```python
from build123d import *

# Parameters (mm, degrees)
F0_W     = 40
F0_H     = 61
F1_DEPTH = 2
F0_H_2   = 19
F2_DEPTH = 25
F3_R     = 8.5
F4_DEPTH = 17
F5_R     = 19.99999


# Not quite as in the source:
# - a fillet or chamfer is up to 0.001 mm smaller than in the source, because OpenCascade refuses the exact size


with BuildPart() as f1:
    # F0 (on Top) → F1 (new body)
    with BuildSketch(Plane.XY):
        with Locations((-2.8480109572, 28.6193176061)):
            Rectangle(F0_W, F0_H)
    extrude(amount=F1_DEPTH)

    # F0 (on Top) → F2 (join)
    with BuildSketch(Plane.XY):
        with Locations((-2.8480109572, -11.3806823939)):
            Rectangle(F0_W, F0_H_2)
    extrude(amount=F2_DEPTH)

    # F3 (on face) → F4 (cut)
    with BuildSketch(Plane(origin=(0, -1.8806823939, 0), x_dir=(-1, 0, 0), z_dir=(0, 1, 0))):
        with Locations((2.8480109572, 13.5)):
            Circle(F3_R)
    extrude(amount=-F4_DEPTH, mode=Mode.SUBTRACT)

    # F5 (radius 20 in the source; OpenCascade refuses exactly that, so slightly less here)
    f5_edges = [f1.edges().sort_by_distance(p)[0] for p in [
        (17.151989, -11.380682, 25),
        (-22.848011, -11.380682, 25),
    ]]
    fillet(f5_edges, radius=F5_R)


solid = f1.part
```
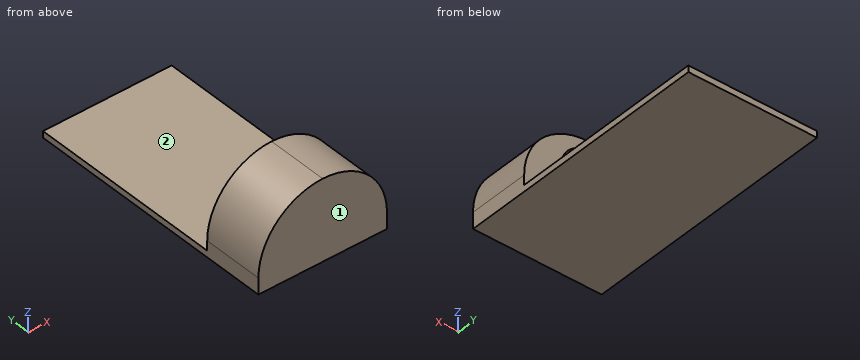
Part model, mm, in its own coordinate system. Face numbers are marked on the shaded views. A direction names the side the tool comes from. Coordinates: 2 decimals unless noted, no trailing zeros. Loops run counter-clockwise (first coordinate to the right, second up) from the corner with the lowest first, then second, coordinate; pieces in that order, holes last. Notation, with made-up numbers: (13.25, 47) - (44.25, 47) arc R11 cw to (44.25, 66) - close; hole circle Ø7 at (51.5, -31). An arc over 180 degrees is marked (long way). Write item = value, one per line. Start each with the question number.
Item 1: 3-axis set-ups, long thin cutter, end or side, ignore diameter. For the marked faces 1 and 2: which of +Z, -Z, +X, -X, +Y, -Y reach the whole face in a straight line?
Item 2: Cut at C-C, the plane y = 12.5. Give the cut face in (x, z), and give its area (3 significant figures).
Item 3: Cut at D-D, the plane z = 11.25. Give the cut face in (x, y).
Item 4: Cut at B-B, the plane x = 1.5. Give the cut face in (y, z).
Item 5: Wall check: L1, parallel to Y at x = -2, z = 11.75; L2, parallel to Y at x = -17, z = 11.25; L3, parallel to Z at x = -11, y = 14. Give the ranges that are in metal, low to high. Write a range as from..to.
Item 6: Flat gauge pins, fed straight in: pin 1 Ø13.5 at (x, z) = (-0.5, 15.5) entering from +Y; pin 2 Ø1 at (x, y) = (-14.5, 36) entering from +Z; pin 3 Ø12 at (x, y) = (4.5, -10.5) entering from +Z. Where does each tip first touch, or does it go through?
The answers:
q1.face_1 = +Z, -Z, +X, -X, -Y
q1.face_2 = +Z, +X, -X, +Y
q2.outline = (-22.85, 0) - (17.15, 0) - (17.15, 2) - (-22.85, 2) - close
q2.area = 80.0 mm2
q3.outline = (-21.85, -20.88) - (16.15, -20.88) - (16.15, -1.88) - (5.35, -1.88) - (5.35, -18.88) - (-11.04, -18.88) - (-11.04, -1.88) - (-21.85, -1.88) - close
q4.outline = (-20.88, 0) - (59.12, 0) - (59.12, 2) - (-1.88, 2) - (-1.88, 6.2) - (-18.88, 6.2) - (-18.88, 20.8) - (-1.88, 20.8) - (-1.88, 24.52) - (-20.88, 24.52) - close
q5.L1 = -20.88..-18.88
q5.L2 = -20.88..-1.88
q5.L3 = 0..2
q6.pin_1 = -1.88
q6.pin_2 = 2
q6.pin_3 = 24.95
